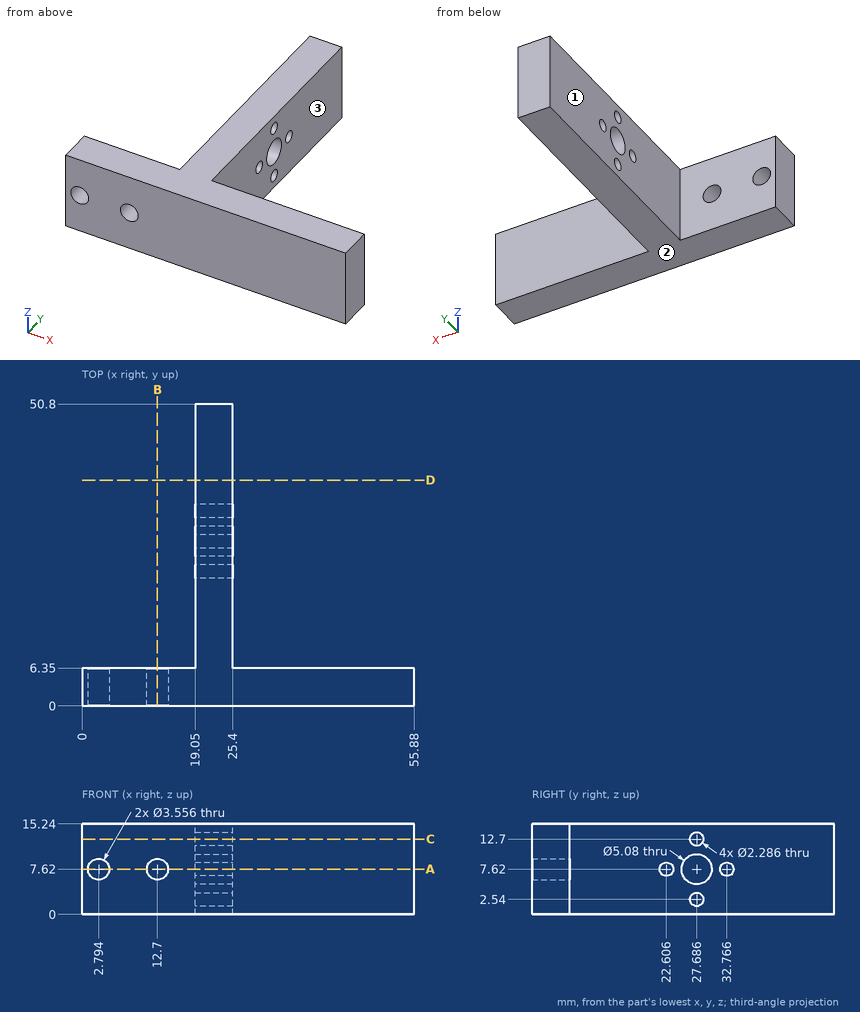
Design review of the part shown in the three views and the two pictorial views. Dimensions are in mm from the part's minimum x, y and z. A direction names the side the tool comes from. Coordinates: 2 decimals unless noted, no trailing zeros. Loops run counter-clockwise (first coordinate to the right, second up) from the corner with the lowest first, then second, coordinate; pieces in that order, holes last.
(1) Insertion check: P1, Ø3, axis at y = 22.606, z = 7.62, coming from the +X side; P2, Ø4, axis at x = 2.794, z = 7.62, coming from the +Y side; P3, Ø4.5, axis at y = 27, z = 10.5, coming from the -X side. Each pin has a flat end and moves straight along its axis. Give the tip position at first contact, or say it passes through.
Determined:
P1: stops at x = 25.4
P2: stops at y = 6.35
P3: stops at x = 19.05
(2) Consider section A-A, the plane z = 7.62. Give the boundary of the cut face in (x, y).
Determined:
outline: (0, 0) - (1.02, 0) - (1.02, 6.35) - (0, 6.35) - close; (4.57, 0) - (10.92, 0) - (10.92, 6.35) - (4.57, 6.35) - close; (14.48, 0) - (55.88, 0) - (55.88, 6.35) - (25.4, 6.35) - (25.4, 21.46) - (19.05, 21.46) - (19.05, 6.35) - (14.48, 6.35) - close; (19.05, 23.75) - (25.4, 23.75) - (25.4, 25.15) - (19.05, 25.15) - close; (19.05, 30.23) - (25.4, 30.23) - (25.4, 31.62) - (19.05, 31.62) - close; (19.05, 33.91) - (25.4, 33.91) - (25.4, 50.8) - (19.05, 50.8) - close
(3) Consider section C-C, the plane z = 12.7. Give the boundary of the cut face in (x, y).
Determined:
outline: (0, 0) - (55.88, 0) - (55.88, 6.35) - (25.4, 6.35) - (25.4, 26.54) - (19.05, 26.54) - (19.05, 6.35) - (0, 6.35) - close; (19.05, 28.83) - (25.4, 28.83) - (25.4, 50.8) - (19.05, 50.8) - close
(4) Tool access review of the marked faces 1, 2 and 3: name each direction out of +Z, -Z, +X, -X, +Y, -Y from which nothing blocks a thin tool from reaching the whole face with its end or side.
Determined:
face 1: +Z, -Z, -X, +Y
face 2: -Z, +X, -X, +Y, -Y
face 3: +Z, -Z, +X, +Y
(5) Wall thickness on L1, parallel to X at y = 3.25, z = 7.62; L2, parallel to Y at x = 22, z = 7.62; L3, parallel to Y at x = 23.5, z = 2.54: over which ranges is each line inside the solid? List them lowest first.
Determined:
L1: x = 0 to 1.02, 4.57 to 10.92, 14.48 to 55.88
L2: y = 0 to 21.46, 23.75 to 25.15, 30.23 to 31.62, 33.91 to 50.8
L3: y = 0 to 26.54, 28.83 to 50.8
(6) Consider section B-B, the plane x = 12.7. Give the boundary of the cut face in (y, z), plus the area to 3 significant figures.
Determined:
outline: (0, 0) - (6.35, 0) - (6.35, 5.84) - (0, 5.84) - close; (0, 9.4) - (6.35, 9.4) - (6.35, 15.24) - (0, 15.24) - close
area: 74.2 mm2
(7) Consider section D-D, the plane y = 38. Give the boundary of the cut face in (x, z), plus the area to 3 significant figures.
Determined:
outline: (19.05, 0) - (25.4, 0) - (25.4, 15.24) - (19.05, 15.24) - close
area: 96.8 mm2
